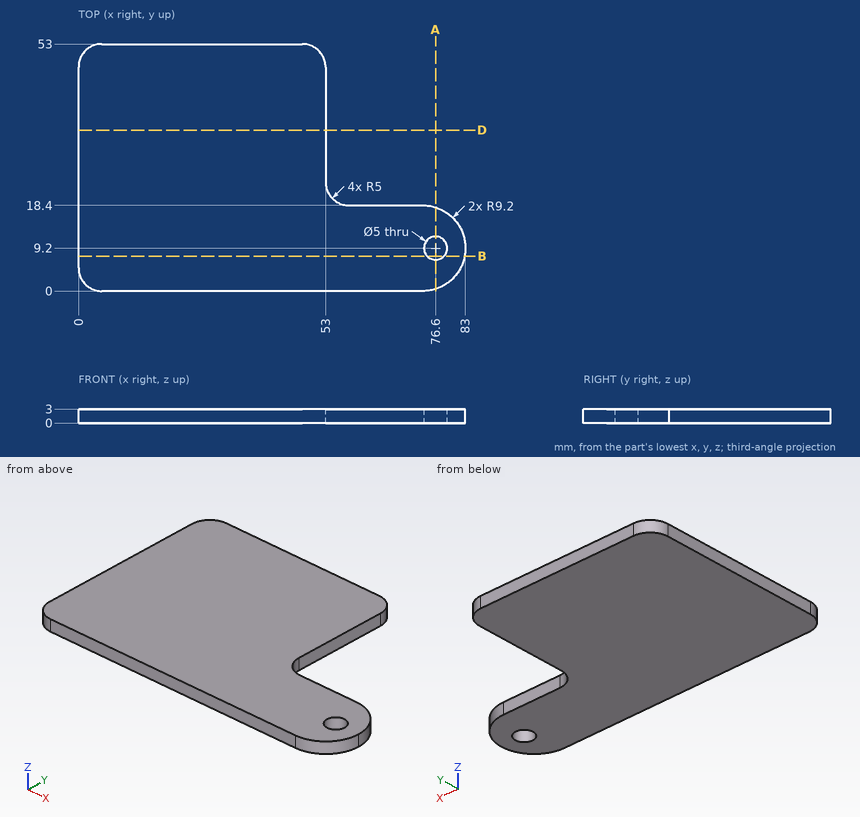
Input: dimensioned drawing with shaded views. Units: mm. Origin: part minimum x, y, z. Coordinates: 2 decimals unless noted, no trailing zeros. Loops run counter-clockwise (first coordinate to the right, second up) from the corner with the lowest first, then second, coordinate; pieces in that order, holes last. Notation, with made-up numbers: (57, 62) -> (97, 62) arc R18 cw to (97, 83) -> close; hole circle Ø6 at (4.5, -23.5). An arc over 180 degrees is marked (long way). One line per item, written item: value. Start each with the question number.
Q1. Section query D-D, the plane y = 34.5. Return the cut outline in (x, z).
Q2. Line query: line 1 along Y through (x, z) = (76.6, 2.3); line 2 along X through (y, z) = (10, 1.1) (1 decimal); line 3 along X through (y, z) = (10.5, 2.8) (1 decimal). Output: solid intervals per line, ascending.
Q3. Section query B-B, the plane y = 7.5. Return the cut outline in (x, z).
Q4. Section query A-A, the plane x = 76.6. Return the cut outline in (y, z), and give its area (3 significant figures).
Q5. Contact query for flat-ended pins moving along their axis: P1, Ø4.5, axis at x = 76.6, y = 9.2, coming from the -Z side; P2, Ø1.5, axis at x = 66, z = 1, coming from the +Y side. Output: stop coordinate, or through.
Results:
1. outline: (0, 0) -> (53, 0) -> (53, 3) -> (0, 3) -> close
2. line 1: 0.44 to 6.7, 11.7 to 17.96
2. line 2: 0 to 74.2, 79 to 83
2. line 3: 0 to 74.5, 78.7 to 82.9
3. outline: (0, 0) -> (74.77, 0) -> (74.77, 3) -> (0, 3) -> close; (78.43, 0) -> (82.84, 0) -> (82.84, 3) -> (78.43, 3) -> close
4. outline: (0.44, 0) -> (6.7, 0) -> (6.7, 3) -> (0.44, 3) -> close; (11.7, 0) -> (17.96, 0) -> (17.96, 3) -> (11.7, 3) -> close
4. area: 37.6 mm^2
5. P1: through
5. P2: y = 18.4
